Work out the finished part from the listing and answer in its coordinate system (mm). Coordinates: 2 decimals unless noted, no trailing zeros. Loops run counter-clockwise (first coordinate to the right, second up) from the corner with the lowest first, then second, coordinate; pieces in that order, holes last. Notation, with made-up numbers: (12.5, 16.25) -> (29.5, 16.25) arc R20 cw to (29.5, 21.25) -> close; hole circle Ø6 at (84.25, 33). An arc over 180 degrees is marked (long way). Use a Markdown table: item, result. Add a question column.
```python
from build123d import *

# Parameters (mm, degrees)
F0_W     = 30
F0_H     = 3
F0_W_2   = 3
F0_H_2   = 30
F1_DEPTH = 3
F2_W     = 3
F2_H     = 30
F3_DEPTH = 25


with BuildPart() as f1:
    # F0 (on Right) → F1 (new body)
    with BuildSketch(Plane.YZ):
        Polygon((0, 67), (0, 0), (68.5, 0), (98.5, 0), (167, 0), (167, 88.5), (167, 118.5), (167, 143.5), (106, 143.5), (106, 67), align=None)
        with Locations((83.5, -1.5)):
            Rectangle(F0_W, F0_H)
        with Locations((168.5, 103.5)):
            Rectangle(F0_W_2, F0_H_2)
    extrude(amount=F1_DEPTH)

    # F2 (on face) → F3 (cut)
    with BuildSketch(Plane.YZ.offset(3)):
        with Locations((107.5, 103.5)):
            Rectangle(F2_W, F2_H)
    extrude(amount=-F3_DEPTH, mode=Mode.SUBTRACT)


solid = f1.part
```
Item 1: Section B-B (y = 124.5) is taken. Determine the outline of the cut face in (x, z), then the cut area to 4 significant figures.
Item 2: Find the intervals of material crossed by probe 1 along Y at (x, z) = (2.7, 12); probe 2 along Z at (x, y) = (1.65, 44); probe 3 along Z at (x, y) = (1.5, 146), in increasing order.
Item 3: Section C-C (z = 81.5) is taken. Determine the outline of the cut face in (x, y).
Item 4: Section A-A (x = 0.7) is taken. Determine the outline of the cut face in (y, z), then the cut area to 3 significant figures.
Item 5: Given pin 1 (0.9 mm diameter, centred on x = 1, y = 168.5, fed in from -Z); pin 2 (6 mm diameter, centred on y = 101, z = 22, fed in from -X); pin 3 (0.9 mm diameter, centred on x = 1, z = 81.5, fed in from -Y); pin 4 (1.5 mm diameter, centred on x = 1.5, z = -1, fed in from -Y), each flat-ended and moving along its own axis, determine where each tip first touches the part or whether it passes through.
Output:
| question | item | result |
|---|---|---|
| 1 | outline | (0, 0) -> (3, 0) -> (3, 143.5) -> (0, 143.5) -> close |
| 1 | area | 430.5 mm2 |
| 2 | probe 1 | y = 0 to 167 |
| 2 | probe 2 | z = 0 to 67 |
| 2 | probe 3 | z = 0 to 143.5 |
| 3 | outline | (0, 106) -> (3, 106) -> (3, 167) -> (0, 167) -> close |
| 4 | outline | (0, 0) -> (68.5, 0) -> (68.5, -3) -> (98.5, -3) -> (98.5, 0) -> (167, 0) -> (167, 88.5) -> (170, 88.5) -> (170, 118.5) -> (167, 118.5) -> (167, 143.5) -> (106, 143.5) -> (106, 118.5) -> (109, 118.5) -> (109, 88.5) -> (106, 88.5) -> (106, 67) -> (0, 67) -> close |
| 4 | area | 15,900 mm2 |
| 5 | pin 1 | stops at z = 88.5 |
| 5 | pin 2 | stops at x = 0 |
| 5 | pin 3 | stops at y = 106 |
| 5 | pin 4 | stops at y = 68.5 |
